For this review, take the finished solid that the model builds, in its own axes (mm). Face numbers are marked on the shaded views. A direction names the side the tool comes from. Round coordinates to 2 decimals unless told otherwise and drop trailing zeros. Order: outer loops, then holes, each group sorted by start corner. A loop starts at its lowest first (then second) coordinate and runs counter-clockwise, first axis right, second up. Notation, with made-up numbers: (55.5, 85.25) -> (62.5, 85.25) arc R23 ccw to (62.5, 103.25) -> close; hole circle Ø3 at (44, -14). An arc over 180 degrees is marked (long way). Use a Markdown table: item, result. Add a question column.
1) Consider section A-A (x = -25). State the section outline as (y, z) points.
2) Consider section D-D (z = 22.5). State the section outline as (x, y) points.
3) Consider section B-B (y = 8.5). State the section outline as (x, z) points, plus the area to 3 significant figures.
4) Consider section C-C (z = -19). State the section outline as (x, y) points, plus the area to 3 significant figures.
5) Clearance check with flat-ended pins moving along their axes: P1, Ø6, axis at y = -9.5, z = 8.5, coming from the +X side; P2, Ø15, axis at x = 33.5, y = 46, coming from the +Z side; P3, Ø3, axis at y = 59, z = -18.5, coming from the -X side; P4, Ø16, axis at x = -62, z = 10.5, coming from the +Y side. State where each tip first meets the part, or that it passes through.
6) Draft analysis for pull direction Y (two halves, no side actions). For the marked faces 4, 5, 6 and 7, state which applies: pulls with the +Y half, pulls with the -Y half, needs draft (parallel to the pull), parting line crosses it, or undercut.
7) Wall thickness on line 1 along X through (y, z) = (3, 10.5); line 2 along X through (y, z) = (-13, -11); line 3 along X through (y, z) = (8, -18): over which ranges is each line inside the solid? List them lowest first. Write a range as [from, to].
8) Machinability: for the marked faces 1, 2 and 3, which of the approach directions +Z, -Z, +X, -X, +Y, -Y give a long, thin tool a straight path to every point of the face, cutting with its end or side? Answer none if there is none.
```python
from build123d import *

# Parameters (mm, degrees)
SKETCH2_R           = 12
SKETCH2_R_2         = 18
BOSS_EXTRUDE2_DEPTH = 35
BOSS_EXTRUDE5_START = 10
BOSS_EXTRUDE5_DEPTH = 10
FILLET2_R           = 10
SKETCH4_R           = 18
CUT_EXTRUDE1_DEPTH  = 20
CUT_EXTRUDE4_DEPTH  = 20


with BuildPart() as part:
    # Sketch2 → Boss-Extrude2 (new, symmetric)
    with BuildSketch(Plane.XY):
        with BuildLine():
            Line((47.053173242, -26.424193548), (47.053173242, 24.306484253))
            ThreePointArc((47.053173242, 24.306484253), (41.053173242, 73.575806452), (35.053173242, 24.306484253))
            Line((35.053173242, 24.306484253), (35.053173242, -16.424193548))
            Line((35.053173242, -16.424193548), (-7.946826758, -16.424193548))
            Line((-7.946826758, -16.424193548), (-7.946826758, 3.575806452))
            ThreePointArc((-7.946826758, 3.575806452), (-27.946826758, 23.575806452), (-47.946826758, 3.575806452))
            Line((-47.946826758, 3.575806452), (-47.946826758, -16.424193548))
            Line((-47.946826758, -16.424193548), (-67.946826758, -16.424193548))
            Line((-67.946826758, -16.424193548), (-67.946826758, -26.424193548))
            Line((-67.946826758, -26.424193548), (47.053173242, -26.424193548))
        make_face()
        with Locations((-27.946826758, 3.575806452)):
            Circle(SKETCH2_R, mode=Mode.SUBTRACT)
        with Locations((41.053173242, 48.575806452)):
            Circle(SKETCH2_R_2, mode=Mode.SUBTRACT)
    extrude(amount=BOSS_EXTRUDE2_DEPTH, both=True)

    # Sketch3 → Boss-Extrude5 (add)
    with BuildSketch(Plane.XY.offset(-35).offset(BOSS_EXTRUDE5_START)):
        with BuildLine():
            ThreePointArc((35.053173242, 24.306484253), (16.542288051, 43.654779406), (26.150658834, 68.648550766))
            Line((26.150658834, 68.648550766), (-39.868838285, 19.634001903))
            ThreePointArc((-39.868838285, 19.634001903), (-18.959063703, 21.442538533), (-7.946826758, 3.575806452))
            Line((-7.946826758, 3.575806452), (-7.946826758, -16.424193548))
            Line((-7.946826758, -16.424193548), (35.053173242, -16.424193548))
            Line((35.053173242, -16.424193548), (35.053173242, 24.306484253))
        make_face()
    extrude(amount=-BOSS_EXTRUDE5_DEPTH)

    # Fillet2
    fillet2_edges = [part.edges().sort_by_distance(p)[0] for p in [
        (-67.946826758, -21.424193548, 35),
    ]]
    fillet(fillet2_edges, radius=FILLET2_R)

    # Sketch4 → Cut-Extrude1 (cut)
    with BuildSketch(Plane.XY.offset(35)):
        with BuildLine():
            ThreePointArc((35.053173242, 24.306484253), (41.053173242, 23.575806452), (47.053173242, 24.306484253))
            ThreePointArc((47.053173242, 24.306484253), (60.738192927, 33.164771444), (66.053173242, 48.575806452))
            ThreePointArc((66.053173242, 48.575806452), (25.642138234, 68.260826137), (35.053173242, 24.306484253))
        make_face()
        with Locations((41.053173242, 48.575806452)):
            Circle(SKETCH4_R, mode=Mode.SUBTRACT)
    extrude(amount=-CUT_EXTRUDE1_DEPTH, mode=Mode.SUBTRACT)

    # Sketch5 → Cut-Extrude4 (cut)
    with BuildSketch(Plane(origin=(47.053173242, 0, 0), x_dir=(0, 0, -1), z_dir=(1, 0, 0))):
        Polygon((-35, 24.306484253), (-35, -11.424193548), (-15, 24.306484253), align=None)
    extrude(amount=-CUT_EXTRUDE4_DEPTH, mode=Mode.SUBTRACT)


solid = part.part
```
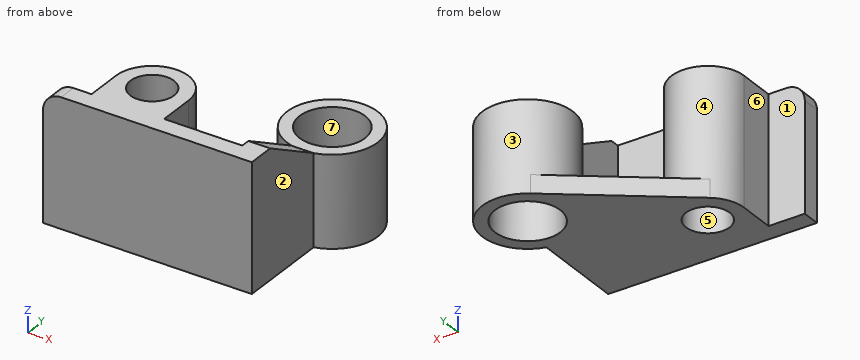
Results list:
| question | item | result |
|---|---|---|
| 1 | outline | (-26.42, -35) -> (-8.06, -35) -> (-8.06, 35) -> (-26.42, 35) -> close; (15.21, -35) -> (30.67, -35) -> (30.67, -25) -> (23.36, -25) -> (23.36, 35) -> (15.21, 35) -> close |
| 2 | outline | (-67.95, -26.42) -> (47.05, -26.42) -> (47.05, 10.91) -> (35.05, 10.91) -> (35.05, -16.42) -> (-7.95, -16.42) -> (-7.95, 3.58) arc R20 ccw to (-47.95, 3.58) -> (-47.95, -16.42) -> (-67.95, -16.42) -> close; hole circle Ø24 at (-27.95, 3.58) |
| 3 | outline | (-47.33, -35) -> (-38.89, -35) -> (-38.89, 35) -> (-47.33, 35) -> close; (-17, -35) -> (47.05, -35) -> (47.05, 23.85) -> (35.05, 23.85) -> (35.05, -25) -> (-8.56, -25) -> (-8.56, 35) -> (-17, 35) -> close |
| 3 | area | 2,320 mm2 |
| 4 | outline | (-67.95, -26.42) -> (47.05, -26.42) -> (47.05, 24.31) arc R25 ccw (long way) to (35.05, 24.31) -> (35.05, -16.42) -> (-7.95, -16.42) -> (-7.95, 3.58) arc R20 ccw to (-47.95, 3.58) -> (-47.95, -16.42) -> (-67.95, -16.42) -> close; hole circle Ø24 at (-27.95, 3.58); hole circle Ø36 at (41.05, 48.58) |
| 4 | area | 3,550 mm2 |
| 5 | P1 | x = 47.05 |
| 5 | P2 | through |
| 5 | P3 | x = 17.7 |
| 5 | P4 | y = -16.42 |
| 6 | face 4 | pulls with the +Y half |
| 6 | face 5 | undercut |
| 6 | face 6 | needs draft |
| 6 | face 7 | undercut |
| 7 | line 1 | [-47.95, -39.93], [-15.96, -7.95], [35.05, 47.05] |
| 7 | line 2 | [-47.95, -7.95], [35.05, 47.05] |
| 7 | line 3 | [-47.45, -39.1], [-16.79, -8.44], [35.05, 47.05] |
| 8 | face 1 | +Z, -Z, -X, +Y |
| 8 | face 2 | +Z, -Z, +X, -Y |
| 8 | face 3 | +Z |
